Source: CAD feature listing. Evaluate the final solid. Frame: model axes, mm. Face numbers are marked on the shaded views. A direction names the side the tool comes from. Coordinates: 2 decimals unless noted, no trailing zeros. Order: outer loops, then holes, each group sorted by start corner. A loop starts at its lowest first (then second) coordinate and runs counter-clockwise, first axis right, second up. Notation, with made-up numbers: (87.25, 63.5) -> (121.25, 63.5) arc R22 ccw to (121.25, 71.5) -> close; hole circle Ø9 at (29.5, -32). An arc over 180 degrees is marked (long way). Put each result on its own line as item: value.
from build123d import *

# Parameters (mm, degrees)
SKETCH1_W           = 108
SKETCH1_H           = 88
BOSS_EXTRUDE2_DEPTH = 2
SKETCH1_3_W         = 112
SKETCH1_3_H         = 92
SKETCH1_3_W_2       = 108
SKETCH1_3_H_2       = 88
BOSS_EXTRUDE3_DEPTH = 26
SKETCH5_W           = 92
SKETCH5_H           = 26
CUT_EXTRUDE1_DEPTH  = 2
SKETCH6_R           = 2.75
CUT_EXTRUDE2_DEPTH  = 1
SKETCH7_R           = 2.5
CUT_EXTRUDE3_DEPTH  = 1
FILLET1_R           = 2
FILLET2_R           = 2
SKETCH9_W           = 38
SKETCH9_H           = 20
CUT_EXTRUDE4_DEPTH  = 2
SKETCH10_W          = 92
SKETCH10_H          = 26
CUT_EXTRUDE5_DEPTH  = 2
FILLET3_R           = 10
FILLET4_R           = 10
FILLET5_R           = 10
SKETCH11_W          = 14
SKETCH11_H          = 88
CUT_EXTRUDE6_DEPTH  = 2


with BuildPart() as part:
    # Sketch1 → Boss-Extrude2 (new body)
    with BuildSketch(Plane(origin=(0, 0, 0), x_dir=(1, 0, 0), z_dir=(0, 1, 0))):
        with Locations((54, 44)):
            Rectangle(SKETCH1_W, SKETCH1_H)
    extrude(amount=BOSS_EXTRUDE2_DEPTH)

    # Sketch1<3> → Boss-Extrude3 (add)
    with BuildSketch(Plane(origin=(0, 0, 0), x_dir=(1, 0, 0), z_dir=(0, 1, 0))):
        with Locations((54, 44)):
            Rectangle(SKETCH1_3_W, SKETCH1_3_H)
        with Locations((54, 44)):
            Rectangle(SKETCH1_3_W_2, SKETCH1_3_H_2, mode=Mode.SUBTRACT)
    extrude(amount=BOSS_EXTRUDE3_DEPTH)

    # Sketch5 → Cut-Extrude1 (cut)
    with BuildSketch(Plane(origin=(110, 0, 0), x_dir=(0, 0, -1), z_dir=(1, 0, 0))):
        with Locations((44, 13)):
            Rectangle(SKETCH5_W, SKETCH5_H)
    extrude(amount=-CUT_EXTRUDE1_DEPTH, mode=Mode.SUBTRACT)

    # Sketch6 → Cut-Extrude2 (cut)
    with BuildSketch(Plane(origin=(0, 0, 0), x_dir=(-1, 0, 0), z_dir=(0, 0, -1))):
        with Locations((-102, 17)):
            Circle(SKETCH6_R)
    extrude(amount=-CUT_EXTRUDE2_DEPTH, mode=Mode.SUBTRACT)

    # Sketch7 → Cut-Extrude3 (cut)
    with BuildSketch(Plane.XY.offset(-88)):
        with Locations((102, 17)):
            Circle(SKETCH7_R)
    extrude(amount=-CUT_EXTRUDE3_DEPTH, mode=Mode.SUBTRACT)

    # Fillet1
    # the kernel refuses this fillet: 2 mm, written as the material it adds along each edge
    with BuildSketch(Plane(origin=(102, 17, 1), x_dir=(-1, 0, 0), z_dir=(0, -1, 0))) as fillet1_piece_1:
        with BuildLine():
            CenterArc((1.017949192, 2), FILLET1_R, 270, 60)
            Line((1.017949192, 0), (1.017949192, -0.04))
            Line((1.017949192, -0.04), (2.75, -0.04))
            Line((2.75, -0.04), (2.79, 0))
            ThreePointArc((2.79, 0), (2.79, 0.5), (2.784641016, 0.98))
            Line((2.784641016, 0.98), (2.75, 1))
        make_face()
    revolve(axis=Axis((102, 17, 1), (0, 0, -1)))

    # Fillet2
    # the kernel refuses this fillet: 2 mm, written as the material it adds along each edge
    with BuildSketch(Plane(origin=(102, 17, -89), x_dir=(1, 0, 0), z_dir=(0, -1, 0))) as fillet2_piece_1:
        with BuildLine():
            CenterArc((0.767949192, 2), FILLET2_R, 270, 60)
            Line((0.767949192, 0), (0.767949192, -0.04))
            Line((0.767949192, -0.04), (2.5, -0.04))
            Line((2.5, -0.04), (2.54, 0))
            ThreePointArc((2.54, 0), (2.54, 0.5), (2.534641016, 0.98))
            Line((2.534641016, 0.98), (2.5, 1))
        make_face()
    revolve(axis=Axis((102, 17, -89), (0, 0, 1)))

    # Sketch9 → Cut-Extrude4 (cut)
    with BuildSketch(Plane.XY.offset(2)):
        with Locations((17, 16)):
            Rectangle(SKETCH9_W, SKETCH9_H)
    extrude(amount=-CUT_EXTRUDE4_DEPTH, mode=Mode.SUBTRACT)

    # Sketch10 → Cut-Extrude5 (cut)
    with BuildSketch(Plane.ZY.offset(2)):
        with Locations((-44, 13)):
            Rectangle(SKETCH10_W, SKETCH10_H)
    extrude(amount=-CUT_EXTRUDE5_DEPTH, mode=Mode.SUBTRACT)

    # Fillet3
    fillet3_edges = [part.edges().sort_by_distance(p)[0] for p in [
        (36, 26, 1),
    ]]
    fillet(fillet3_edges, radius=FILLET3_R)

    # Fillet4
    fillet4_edges = [part.edges().sort_by_distance(p)[0] for p in [
        (108, 26, 1),
    ]]
    fillet(fillet4_edges, radius=FILLET4_R)

    # Fillet5
    fillet5_edges = [part.edges().sort_by_distance(p)[0] for p in [
        (108, 26, -89),
    ]]
    fillet(fillet5_edges, radius=FILLET5_R)

    # Sketch11 → Cut-Extrude6 (cut)
    with BuildSketch(Plane(origin=(0, 0, 0), x_dir=(-1, 0, 0), z_dir=(0, -1, 0))):
        with Locations((-101, 44)):
            Rectangle(SKETCH11_W, SKETCH11_H)
    extrude(amount=-CUT_EXTRUDE6_DEPTH, mode=Mode.SUBTRACT)


solid = part.part
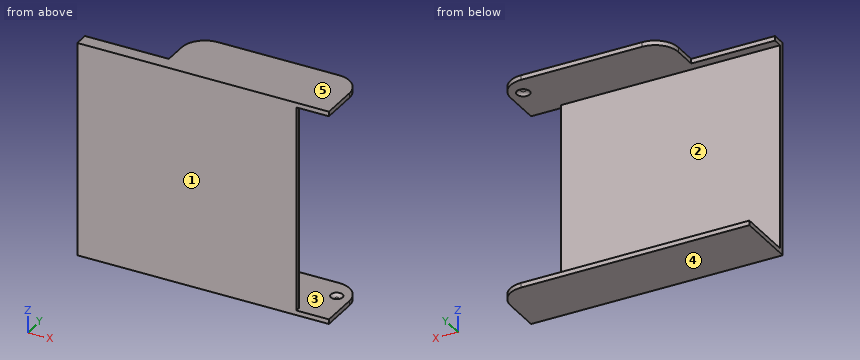
1. Cut plane B-B on x = 14.5. Output: boundary loops of the cut face in (y, z).
Numbers:
outline: (0, -90) -> (26, -90) -> (26, -88) -> (2, -88) -> (2, 0) -> (6, 0) -> (6, 2) -> (0, 2) -> close
2. Ray query, line 1 along Z through (x, y) = (19.5, 5); line 2 along Y through (x, z) = (21, -60); line 3 along Z through (x, y) = (16, 9.5). Return the intervals inside material, ascending.
Numbers:
line 1: z = -90 to -88, 0 to 2
line 2: y = 0 to 2
line 3: z = -90 to -88
3. Cut plane A-A on y = 23.25. Output: boundary loops of the cut face in (x, z).
Numbers:
outline: (0, -90) -> (104.89, -90) -> (104.89, -88) -> (0, -88) -> close; (39.11, 0) -> (104.89, 0) -> (104.89, 2) -> (39.11, 2) -> close
4. First-contact query: pin 1 (5 mm diameter, centred on y = 6, z = -27.5, fed in from -X); pin 2 (2 mm diameter, centred on x = 91, z = -76, fed in from +Y); pin 3 (1.6 mm diameter, centred on x = 12.5, z = 1, fed in from +Y); pin 4 (0.6 mm diameter, centred on y = 12.5, z = 1.5, fed in from -X). Flat tips, straight axial feed; report the tip coordinate or a pass-through.
Numbers:
pin 1: passes through
pin 2: stops at y = 2
pin 3: stops at y = 6
pin 4: stops at x = 36
5. Cut plane D-D on z = -32. Output: boundary loops of the cut face in (x, y).
Numbers:
outline: (0, 0) -> (94, 0) -> (94, 2) -> (0, 2) -> close
6. Pull-direction query (Z, two-part tool) for the marked faces 3, 4 and 5; classes: pulls with the +Z half, pulls with the -Z half, needs draft (parallel to the pull), parting line crosses it, or undercut.
Numbers:
face 3: undercut
face 4: pulls with the -Z half
face 5: pulls with the +Z half
7. Set-up query: the marked faces 1 and 2. Return all of +Z, -Z, +X, -X, +Y, -Y with unobstructed straight access to the full face (end or side cutting, diameter ignored); none if empty.
Numbers:
face 1: +Z, -Z, +X, -X, -Y
face 2: +X, -X, +Y
8. Cut plane C-C on y = 13. Output: boundary loops of the cut face in (x, z), plus the area to 3 significant figures.
Numbers:
outline: (0, -90) -> (108, -90) -> (108, -88) -> (0, -88) -> close; (36, 0) -> (108, 0) -> (108, 2) -> (36, 2) -> close
area: 360 mm2
